Input: part model. Units: mm. Frame: model coordinates. A direction names the side the tool comes from. Round coordinates to 2 decimals unless told otherwise and drop trailing zeros. Loops run counter-clockwise (first coordinate to the right, second up) from the corner with the lowest first, then second, coordinate; pieces in that order, holes last. Notation, with made-up numbers: M 64,83.5 L 112,83.5 A35 cw 112,118.5 Z; hole C -13.75,-19 d7. An arc over 180 degrees is marked long. Return JSON: item names as keys, results as strings. Group by question number.
1) Section C-C (z = 19). Output: boundary loops of the cut face in (x, y), plus the area to 3 significant figures.
2) Section B-B (x = -10.5). Count the separate pieces of the cut face and the enclosed holes in it, plus the area to 3 significant figures.
3) Contact query for flat-ended pins moving along their axis: P1, Ø8, axis at x = -8, y = -10, coming from the +Z side; P2, Ø8, axis at x = -10.23, y = 65.64, coming from the +Z side; P3, Ø3.5, axis at x = -85.23, y = -9.36, coming from the -Z side; P4, Ø1.5, axis at y = 1, z = 16.5, coming from the +X side. Output: stop coordinate, or through.
4) Mould query, pull axis X, two halves, no side actions, for faces 3 (the face through (-7.195, 40.902, 15.231)), 4 (the face through (-8, -12, 4)), 5 (the face through (-2.733, 28, 5)). Classes: +X half, -X half, draft (parallel to the pull), parting line (faces both ways), or undercut.
5) Section D-D (z = 24.75). Output: boundary loops of the cut face in (x, y), plus the area to 3 significant figures.
6) Section A-A (z = 5.25). Output: boundary loops of the cut face in (x, y).
7) Material intervals for line 1 (Y direction, x = -49, z = 20.25); line 2 (Z direction, x = -76, y = -11); line 3 (X direction, y = 26, z = 16), sorted ascending. Write a range as from..to.
8) Access query for faces 1 (the face through (-83, 63, 4)), 2 (the face through (-9.84, 62.66, 2.03)). Directions: +Z, -Z, +X, -X, +Y, -Y. A direction counts if a zero-diameter tool reaches every point of the face in a straight line with its end or side. Return the directions, or none.
from build123d import *

# Parameters (mm, degrees)
SKETCH_1_W          = 90
SKETCH_1_H          = 90
EXTRUDE_3_DEPTH     = 10
SKETCH_3_R          = 35
CUT_EXTRUDE_2_DEPTH = 10
EXTRUDE_START       = 20
SKETCH_4_R          = 42.5
SKETCH_4_R_2        = 35
EXTRUDE_4_DEPTH     = 20
FILLET_1_R          = 10
SKETCH_5_R          = 3
CUT_EXTRUDE_3_DEPTH = 10
SKETCH_6_R          = 5
CUT_EXTRUDE_4_DEPTH = 6


with BuildPart() as part:
    # 스케치1 → 보스-돌출3 (new body)
    with BuildSketch(Plane.XY):
        with Locations((-47.732849402, 28.135926797)):
            Rectangle(SKETCH_1_W, SKETCH_1_H)
    extrude(amount=EXTRUDE_3_DEPTH)

    # 스케치3 → 컷-돌출2 (cut)
    with BuildSketch(Plane.XY.offset(10)):
        with Locations((-47.732849402, 28.135926797)):
            Circle(SKETCH_3_R)
    extrude(amount=-CUT_EXTRUDE_2_DEPTH, mode=Mode.SUBTRACT)

    # 스케치4 → 보스-돌출4 (add)
    with BuildSketch(Plane.XY.offset(10).offset(EXTRUDE_START)):
        with Locations((-47.732849402, 28.135926797)):
            Circle(SKETCH_4_R)
        with Locations((-47.732849402, 28.135926797)):
            Circle(SKETCH_4_R_2, mode=Mode.SUBTRACT)
    extrude(amount=-EXTRUDE_4_DEPTH)

    # 필렛1
    # the kernel refuses this fillet: 10 mm, written as the material it takes off along each edge
    with BuildSketch(Plane(origin=(-47.732849402, 28.135926797, 30), x_dir=(1, 0, 0), z_dir=(0, -1, 0))) as fillet_1_piece_1:
        with BuildLine():
            CenterArc((32.5, -9.682458366), FILLET_1_R, 0, 75.522487814)
            Line((35, 0), (35.05, 0.193649167))
            ThreePointArc((35.05, 0.193649167), (38.75, 0.2), (42.5, 0.2))
            Line((42.5, 0.2), (42.7, 0))
            Line((42.7, 0), (42.7, -9.682458366))
            Line((42.7, -9.682458366), (42.5, -9.682458366))
        make_face()
    revolve(axis=Axis((-47.732849402, 28.135926797, 30), (0, 0, 1)), mode=Mode.SUBTRACT)

    # 스케치5 → 컷-돌출3 (cut)
    with BuildSketch(Plane.XY.offset(10)):
        with Locations((-85.232849402, 65.635926797)):
            Circle(SKETCH_5_R)
        with Locations(Location((-10.232849402, 65.635926797, 0), (0, 0, 180))):
            Circle(SKETCH_5_R)
        with Locations((-10.232849402, -9.364073203)):
            Circle(SKETCH_5_R)
        with Locations(Location((-85.232849402, -9.364073203, 0), (0, 0, 180))):
            Circle(SKETCH_5_R)
    extrude(amount=-CUT_EXTRUDE_3_DEPTH, mode=Mode.SUBTRACT)

    # 스케치6 → 컷-돌출4 (cut)
    with BuildSketch(Plane.XY.offset(10)):
        with Locations((-85.232849402, 65.635926797)):
            Circle(SKETCH_6_R)
        with Locations(Location((-10.232849402, 65.635926797, 0), (0, 0, 180))):
            Circle(SKETCH_6_R)
        with Locations((-10.232849402, -9.364073203)):
            Circle(SKETCH_6_R)
        with Locations(Location((-85.232849402, -9.364073203, 0), (0, 0, 180))):
            Circle(SKETCH_6_R)
    extrude(amount=-CUT_EXTRUDE_4_DEPTH, mode=Mode.SUBTRACT)


solid = part.part
Returned:
{
 "1": {"outline": "C -47.73,28.14 d85; hole C -47.73,28.14 d70", "area": "1,830 mm^2"},
 "2": {"separate pieces": "3", "enclosed holes": "0", "area": "1,450 mm^2"},
 "3": {"P1": "stops at z = 10", "P2": "stops at z = 4", "P3": "passes through", "P4": "stops at x = -14.42"},
 "4": {"face 3": "parting line", "face 4": "undercut", "face 5": "+X half"},
 "5": {"outline": "C -47.73,28.14 d82.93; hole C -47.73,28.14 d70", "area": "1,550 mm^2"},
 "6": {"outline": "M -92.73,-16.86 L -2.73,-16.86 L -2.73,73.14 L -92.73,73.14 Z; hole C -85.23,-9.36 d10; hole C -85.23,65.64 d10; hole C -47.73,28.14 d70; hole C -10.23,-9.36 d10; hole C -10.23,65.64 d10"},
 "7": {"line 1": "y = -14.35..-6.84, 63.11..70.62", "line 2": "z = 0..10", "line 3": "x = -90.18..-82.67, -12.8..-5.29"},
 "8": {"face 1": "+Z", "face 2": "+Z, -Z"}
}
